Can you work these out from the model? Positions are in its coordinate system, mm. A direction names the side the tool comes from. Coordinates: 2 decimals unless noted, no trailing zeros. Loops run counter-clockwise (first coordinate to the right, second up) from the corner with the lowest first, then second, coordinate; pieces in that order, holes last. Notation, with made-up numbers: (47, 41.5) -> (92, 41.5) arc R12 cw to (92, 50.5) -> close; hole circle Ø4 at (42, 22). An arc over 180 degrees is marked (long way). Put each result on its own line as item: value. Start each with the question number.
Item 1: For faces 4 (the flat face through (0, 3, -5)), 5 (the flat face through (0, -2.5, 0)), which set-ups out of +Z, -Z, +X, -X, +Y, -Y let a thin tool reach every point of the face, with its end or its side?
Item 2: We'd pull the mould along Y, two halves only. Please class faces 1 (the flat face through (0, 0, 5)), 2 (the cylindrical face through (-5, 0, 10)), 3 (the flat face through (0, 0, 25)): pulls with the +Y half, pulls with the -Y half, needs draft (parallel to the pull), parting line crosses it, or undercut.
Item 3: If we section it at C-C on z = 18.5: Please give me the cut outline in (x, y), plus the area to 3 significant figures.
Item 4: Please list where these lines run through material, in increasing order: L1, parallel to Y at x = -0.25, z = -2.25; L2, parallel to Z at x = -1.5, y = -2.25; L3, parallel to Y at x = -2.5, z = 2. Write a range as from..to.
Item 5: If we section it at B-B on y = 0: Please give me the cut outline in (x, z).
Item 6: If we section it at A-A on x = 0: Please give me the cut outline in (y, z).
Item 7: Will these pins go through, and if not, where does the flat tip stop? P1, Ø2, axis at y = -3, z = 20, coming from the +X side; P2, Ø2, axis at x = 1.5, z = -2, coming from the -Y side.
Item 8: If we section it at D-D on x = 4: Please give me the cut outline in (y, z).
```python
from build123d import *

# Parameters (mm, degrees)
SKETCH1_R                = 5
BOSS_EXTRUDE1_DEPTH      = 25
BOSS_EXTRUDE1_DEPTH_BACK = 5
SKETCH3_W                = 10
SKETCH3_H                = 5
CUT_EXTRUDE2_DEPTH       = 6
CUT_EXTRUDE2_DEPTH_BACK  = 6


with BuildPart() as part:
    # Sketch1 → Boss-Extrude1 (new body, two sides)
    with BuildSketch(Plane.XY) as boss_extrude1_sk:
        Circle(SKETCH1_R)
    extrude(amount=BOSS_EXTRUDE1_DEPTH)
    extrude(boss_extrude1_sk.sketch, amount=-BOSS_EXTRUDE1_DEPTH_BACK)

    # Sketch3 → Cut-Extrude2 (cut, two sides)
    with BuildSketch(Plane(origin=(0, 0, 0), x_dir=(0, 0, -1), z_dir=(1, 0, 0))) as cut_extrude2_sk:
        Rectangle(SKETCH3_W, SKETCH3_H)
    extrude(amount=CUT_EXTRUDE2_DEPTH, mode=Mode.SUBTRACT)
    extrude(cut_extrude2_sk.sketch, amount=-CUT_EXTRUDE2_DEPTH_BACK, mode=Mode.SUBTRACT)


solid = part.part
```
Solutions:
1. face 4: -Z, +X, -X, +Y, -Y
1. face 5: -Z, +X, -X
2. face 1: undercut
2. face 2: parting line crosses it
2. face 3: needs draft
3. outline: circle Ø10 at (0, 0)
3. area: 78.5 mm^2
4. L1: -4.99..-2.5, 2.5..4.99
4. L2: 5..25
4. L3: -4.33..-2.5, 2.5..4.33
5. outline: (-5, 5) -> (5, 5) -> (5, 25) -> (-5, 25) -> close
6. outline: (-5, -5) -> (-2.5, -5) -> (-2.5, 5) -> (2.5, 5) -> (2.5, -5) -> (5, -5) -> (5, 25) -> (-5, 25) -> close
7. P1: x = 4.58
7. P2: y = -4.97
8. outline: (-3, -5) -> (-2.5, -5) -> (-2.5, 5) -> (2.5, 5) -> (2.5, -5) -> (3, -5) -> (3, 25) -> (-3, 25) -> close
